from build123d import *

# Parameters (mm, degrees)
F1_DEPTH = 25
F2_R     = 4.99999


# Not quite as in the source:
# - a fillet or chamfer is up to 0.001 mm smaller than in the source, because OpenCascade refuses the exact size


with BuildPart() as f1:
    # F0 (on Top) → F1 (new body)
    with BuildSketch(Plane.XY):
        Polygon((-35, 0), (0, 0), (0, 45), (22, 45), (22, 55), (-32.3444679379, 55), (-32.3444679379, 45), (-10.3444679379, 45), (-10.3444679379, 10), (-35, 10), align=None)
    extrude(amount=F1_DEPTH)

    # F2 (radius 5 in the source; OpenCascade refuses exactly that, so slightly less here)
    f2_edges = [f1.edges().sort_by_distance(p)[0] for p in [
        (-5.172234, 55, 0),
        (-32.344468, 50, 0),
        (-10.344468, 27.5, 0),
        (-21.344468, 45, 0),
        (11, 45, 0),
        (22, 50, 0),
        (0, 22.5, 0),
        (-17.5, 0, 0),
        (-22.672234, 10, 0),
        (-35, 5, 0),
        (-5.172234, 55, 25),
        (11, 45, 25),
        (-21.344468, 45, 25),
        (-32.344468, 50, 25),
        (22, 50, 25),
        (-10.344468, 27.5, 25),
        (-22.672234, 10, 25),
        (-35, 5, 25),
        (-17.5, 0, 25),
        (0, 22.5, 25),
    ]]
    fillet(f2_edges, radius=F2_R)


solid = f1.part
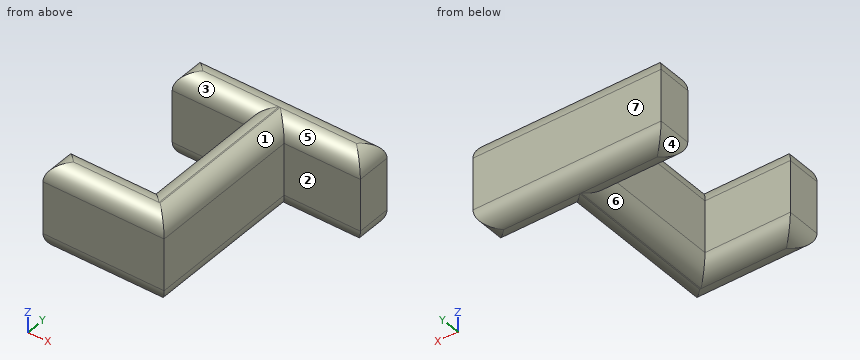
CAD build for the part. Positions are in the model's coordinates, mm. Face numbers are marked on the shaded views. A direction names the side the tool comes from. Coordinates: 2 decimals unless noted, no trailing zeros. Loops run counter-clockwise (first coordinate to the right, second up) from the corner with the lowest first, then second, coordinate; pieces in that order, holes last. Notation, with made-up numbers: (47, 62) - (56, 62) arc R24 cw to (56, 97) - close; hole circle Ø8 at (-10, 40.5). An arc over 180 degrees is marked (long way). Write item = value, one per line. Start each with the question number.
Q1. Pull direction Y, two halves, no side cores. Call the marked faces 5, 6 and 7: pulls with the +Y half, pulls with the -Y half, needs draft (parallel to the pull), parting line crosses it, or undercut.
Q2. Flat gauge pins, fed straight in: pin 1 Ø7.5 at (x, z) = (13, 11) entering from -Y; pin 2 Ø3 at (y, z) = (51, 14) entering from -X; pin 3 Ø4.5 at (y, z) = (29.5, 14.5) entering from +X. Where does each tip first touch, or does it go through?
Q3. Which spindle directions (+Z, -Z, +X, -X, +Y, -Y) get a long thin tool onto all of the face, cutting with end or side? Do the marked faces 1, 2, 3 and 4. Say none if no direction does.
Q4. Cut at B-B, the plane z = 13.5. List the corners of the cut face in (x, y).
Q5. Cut at C-C, the plane y = 21. List the corners of the cut face in (x, z).
Q6. Drill centre lines: L1, parallel to Y at x = -31.5, z = 13; L2, parallel to X at y = 12.5, z = 11.5; L3, parallel to Y at x = 0.5, z = 14.5. Where is each one in solid material? Low to high.
Computed:
q1.face_5 = pulls with the -Y half
q1.face_6 = undercut
q1.face_7 = pulls with the +Y half
q2.pin_1 = 45
q2.pin_2 = -32.34
q2.pin_3 = 0
q3.face_1 = +Z, +X, -Y
q3.face_2 = +Z, -Z, +X, -Y
q3.face_3 = +Z, -X
q3.face_4 = -Z, -X, +Y
q4.outline = (-35, 0) - (0, 0) - (0, 45) - (22, 45) - (22, 55) - (-32.34, 55) - (-32.34, 45) - (-10.34, 45) - (-10.34, 10) - (-35, 10) - close
q5.outline = (-10.34, 5) arc R5 ccw to (-5.34, 0) - (-5, 0) arc R5 ccw to (0, 5) - (0, 20) arc R5 ccw to (-5, 25) - (-5.34, 25) arc R5 ccw to (-10.34, 20) - close
q6.L1 = 0 to 10, 45 to 55
q6.L2 = -10.34 to 0
q6.L3 = 45 to 55
